Here's how the part is built. I have some questions about the finished solid (model axes, mm). A direction names the side the tool comes from. Give positions to 0.01 mm unless a question says otherwise; leave off trailing zeros. Loops run counter-clockwise (first coordinate to the right, second up) from the corner with the lowest first, then second, coordinate; pieces in that order, holes last. Notation, with made-up numbers: (40, 55.5) -> (93, 55.5) arc R23 cw to (93, 90.5) -> close; hole circle Ø6 at (7.25, 9.5). An arc over 180 degrees is marked (long way). Answer in a Markdown table with one row per item. Add a question column.
Item 1: If we section it at B-B (x = 0): Write out the boundary of the cut face in (y, z), then the cut area to 3 significant figures.
Item 2: We'd pull the mould along Z, two halves only. Please class faces 3 (the face through (-15, 0.1, -8.1)), 4 (the face through (18.655, 0.119, -4.143)), 5 (the face through (-9, 0, 14)): released by +Z, released by -Z, zero draft, split by the parting line, or undercut.
Item 3: Which directions (+Z, -Z, +X, -X, +Y, -Y) give clear straight access to the entire face, cutting with the end or side of a thin tool? Please do faces 1 (the face through (-17, 5.9, 9)), 2 (the face through (14.505, 2.016, 7.545)).
Item 4: If we section it at A-A (z = 0): Write out the boundary of the cut face in (x, y), then the cut area to 3 significant figures.
Item 5: For P1, Ø2, axis at x = -8.5, y = 3.5, coming from the -Z side; P2, Ø2, axis at y = 3, z = 12.5, coming from the -X side; P3, Ø3, axis at y = 1.5, z = -7, coming from the +X side, each with a flat end and sliding along its axis, tell me the tip position at first contact or that it passes through.
Item 6: If we section it at C-C (y = 1.2): Write out the boundary of the cut face in (x, z), then the cut area to 3 significant figures.
Item 7: If I drill on line 1 (X direction, y = 5.95, z = 0); line 2 (Z direction, x = 0, y = 2.75); line 3 (Y direction, x = -16.5, z = -9), over which ranges is the centre line in solid material (lowest first)?
```python
from build123d import *

# Parameters (mm, degrees)
SKETCH_3_R          = 20.4
SKETCH_3_R_2        = 18.76
CUT_EXTRUDE_1_DEPTH = 0.1
SKETCH_4_R          = 18.49
SKETCH_4_R_2        = 16.85
CUT_EXTRUDE_2_DEPTH = 0.1


with BuildPart() as part:
    # 草图2 → 旋转1 (revolve)
    with BuildSketch(Plane(origin=(0, 0, 0), x_dir=(0, 0, -1), z_dir=(1, 0, 0))):
        Polygon((-20.9, 1.91), (-20.9, 6), (-18.26, 6), (-16.35, 4.09), (-16.35, 0), (-18.99, 0), align=None)
    revolve(axis=Axis((0, 0, 0), (0, -1, 0)))

    # 草图3 → 切除-拉伸1 (cut)
    with BuildSketch(Plane(origin=(0, 6, 0), x_dir=(1, 0, 0), z_dir=(0, 1, 0))):
        with Locations(Location((0, 0, 0), (0, 0, 270))):
            Circle(SKETCH_3_R)
        with Locations(Location((0, 0, 0), (0, 0, 270))):
            Circle(SKETCH_3_R_2, mode=Mode.SUBTRACT)
    extrude(amount=-CUT_EXTRUDE_1_DEPTH, mode=Mode.SUBTRACT)

    # 草图4 → 切除-拉伸2 (cut)
    with BuildSketch(Plane.XZ):
        with Locations(Location((0, 0, 0), (0, 0, 270))):
            Circle(SKETCH_4_R)
        with Locations(Location((0, 0, 0), (0, 0, 270))):
            Circle(SKETCH_4_R_2, mode=Mode.SUBTRACT)
    extrude(amount=-CUT_EXTRUDE_2_DEPTH, mode=Mode.SUBTRACT)


solid = part.part
```
Recorded:
| question | item | result |
|---|---|---|
| 1 | outline | (0, -18.99) -> (1.91, -20.9) -> (6, -20.9) -> (6, -20.4) -> (5.9, -20.4) -> (5.9, -18.76) -> (6, -18.76) -> (6, -18.26) -> (4.09, -16.35) -> (0, -16.35) -> (0, -16.85) -> (0.1, -16.85) -> (0.1, -18.49) -> (0, -18.49) -> close; (0, 16.35) -> (4.09, 16.35) -> (6, 18.26) -> (6, 18.76) -> (5.9, 18.76) -> (5.9, 20.4) -> (6, 20.4) -> (6, 20.9) -> (1.91, 20.9) -> (0, 18.99) -> (0, 18.49) -> (0.1, 18.49) -> (0.1, 16.85) -> (0, 16.85) -> close |
| 1 | area | 46.6 mm^2 |
| 2 | face 3 | undercut |
| 2 | face 4 | split by the parting line |
| 2 | face 5 | zero draft |
| 3 | face 1 | +Y |
| 3 | face 2 | +Y, -Y |
| 4 | outline | (-20.9, 1.91) -> (-18.99, 0) -> (-18.49, 0) -> (-18.49, 0.1) -> (-16.85, 0.1) -> (-16.85, 0) -> (-16.35, 0) -> (-16.35, 4.09) -> (-18.26, 6) -> (-18.76, 6) -> (-18.76, 5.9) -> (-20.4, 5.9) -> (-20.4, 6) -> (-20.9, 6) -> close; (16.35, 0) -> (16.85, 0) -> (16.85, 0.1) -> (18.49, 0.1) -> (18.49, 0) -> (18.99, 0) -> (20.9, 1.91) -> (20.9, 6) -> (20.4, 6) -> (20.4, 5.9) -> (18.76, 5.9) -> (18.76, 6) -> (18.26, 6) -> (16.35, 4.09) -> close |
| 4 | area | 46.6 mm^2 |
| 5 | P1 | stops at z = -19.51 |
| 5 | P2 | stops at x = -17.45 |
| 5 | P3 | stops at x = 20.15 |
| 6 | outline | circle Ø40.38 at (0, 0); hole circle Ø32.7 at (0, 0) |
| 6 | area | 441 mm^2 |
| 7 | line 1 | x = -20.9 to -20.4, -18.76 to -18.21, 18.21 to 18.76, 20.4 to 20.9 |
| 7 | line 2 | z = -20.9 to -16.35, 16.35 to 20.9 |
| 7 | line 3 | y = 0 to 5.9 |
